Source: CAD feature listing. Evaluate the final solid. Frame: model axes, mm. A direction names the side the tool comes from. Give positions to 0.01 mm unless a question says otherwise; leave off trailing zeros.
1) Material intervals for line 1 (Y direction, x = 354, z = 12.5) (3 decimals); line 2 (Y direction, x = 605, z = 16) (3 decimals); line 3 (Z direction, x = 413, y = 15) (3 decimals), sorted ascending.
2) Access query for faces 1 (the face through (425, 88, 0)), 2 (the face through (825.5, 15, 16)), 3 (the face through (12.7, 15, 16)). Directions: +Z, -Z, +X, -X, +Y, -Y. A direction counts if a zero-diameter tool reaches every point of the face in a straight line with its end or side. Return the directions, or none.
3) First-contact query: P1, Ø12, axis at x = 114.5, y = 82.5, coming from the -Z side; P2, Ø1, axis at x = 533.5, z = 5, coming from the -Y side (3 decimals); P3, Ø10, axis at x = 831, z = 7, coming from the -Y side; P4, Ø6.5, axis at y = 17, z = 11, coming from the -X side. Flat tips, straight axial feed; report the tip coordinate or a pass-through.
```python
from build123d import *

# Parameters (mm, degrees)
F0_W     = 419.1
F0_H     = 152.4
F1_DEPTH = 22.225
F2_W     = 12.7
F2_H     = 25.4
F3_DEPTH = 22.226
F4_W     = 9.525
F4_H     = 11.1125
F5_DEPTH = 419.101


with BuildPart() as f1:
    # F0 (on Top) → F1 (new body)
    with BuildSketch(Plane.XY):
        with Locations((209.55, 76.2)):
            Rectangle(F0_W, F0_H)
    extrude(amount=F1_DEPTH)

    # F2 (on face) → F3 (cut, through all)
    with BuildSketch(Plane.XY.offset(22.225)):
        with Locations((6.35, 12.7)):
            Rectangle(F2_W, F2_H)
    extrude(amount=-F3_DEPTH, mode=Mode.SUBTRACT)

    # F4 (on face) → F5 (cut, through all)
    with BuildSketch(Plane.YZ.offset(419.1)):
        Polygon((12.7, 12.7), (0, 12.7), (0, 0), (22.225, 0), (22.225, 6.35), (12.7, 6.35), align=None)
        with Locations((147.6375, 16.66875)):
            Rectangle(F4_W, F4_H)
    extrude(amount=-F5_DEPTH, mode=Mode.SUBTRACT)

    # F6: F1 across face


with BuildPart() as f1_1:
    add(f1.part)
    add(f1.part.mirror(Plane(origin=(419.1, 78.572096, 11.328264), x_dir=(0, 1, 0), z_dir=(1, 0, 0))))


solid = f1_1.part
```
From the geometry:
1. line 1: y = 12.7 to 142.875
1. line 2: y = 0 to 142.875
1. line 3: z = 6.35 to 22.225
2. face 1: -Z, +X, -X, +Y, -Y
2. face 2: +Z, -Z, +X, -Y
2. face 3: +Z, -Z, -X, -Y
3. P1: stops at z = 0
3. P2: stops at y = 22.225
3. P3: stops at y = 25.4
3. P4: stops at x = 12.7
